Geometry: final body of the model. Coordinates: model frame, mm. Face numbers are marked on the shaded views. A direction names the side the tool comes from. Give positions to 0.01 mm unless a question says otherwise; leave off trailing zeros. Order: outer loops, then holes, each group sorted by start corner. A loop starts at its lowest first (then second) coordinate and runs counter-clockwise, first axis right, second up. Notation, with made-up numbers: (68.5, -38) - (106.5, -38) arc R20 cw to (106.5, -26) - close; hole circle Ø7 at (14.5, -37). An arc over 180 degrees is marked (long way). One line per item, written item: value.
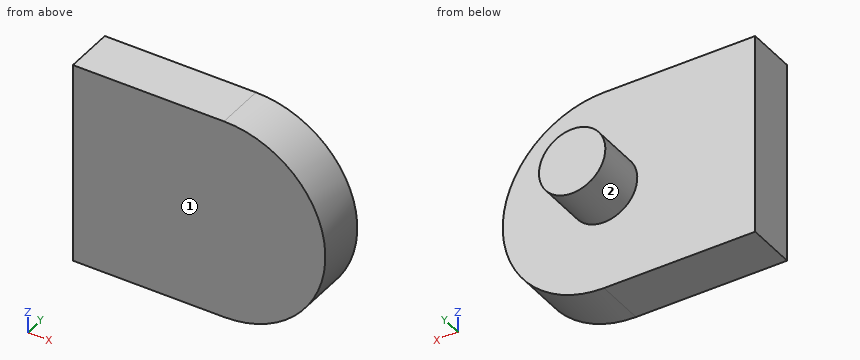
```python
from build123d import *

# Parameters (mm, degrees)
BOSS_EXTRUDE1_DEPTH = 3
SKETCH4_R           = 2
BOSS_EXTRUDE2_DEPTH = 3


with BuildPart() as part:
    # Sketch3 → Boss-Extrude1 (new body)
    with BuildSketch(Plane(origin=(0, 0, 0), x_dir=(1, 0, 0), z_dir=(0, 1, 0))):
        with BuildLine():
            Line((-20.336842105, 8.293859649), (-11.236842105, 8.293859649))
            ThreePointArc((-11.236842105, 8.293859649), (-5.136842105, 2.193859649), (-11.236842105, -3.906140351))
            Line((-11.236842105, -3.906140351), (-20.336842105, -3.906140351))
            Line((-20.336842105, -3.906140351), (-20.336842105, 8.293859649))
        make_face()
    extrude(amount=BOSS_EXTRUDE1_DEPTH)

    # Sketch4 → Boss-Extrude2 (add)
    with BuildSketch(Plane(origin=(0, 3, 0), x_dir=(1, 0, 0), z_dir=(0, 1, 0))):
        with Locations(Location((-11.236842105, 2.193859649, 0), (0, 0, 270))):
            Circle(SKETCH4_R)
    extrude(amount=BOSS_EXTRUDE2_DEPTH)


solid = part.part
```
1) Section A-A, the plane z = -3. Return loops of the section in (x, y), then the cut area to 3 significant figures.
Answers below:
outline: (-20.34, 0) - (-5.19, 0) - (-5.19, 3) - (-9.41, 3) - (-9.41, 6) - (-13.07, 6) - (-13.07, 3) - (-20.34, 3) - close
area: 56.4 mm^2
2) Set-up query: the marked faces 1 and 2. Return all of +Z, -Z, +X, -X, +Y, -Y with unobstructed straight access to the full face (end or side cutting, diameter ignored); none if empty.
Answers below:
face 1: +Z, -Z, +X, -X, -Y
face 2: +Y
3) Section C-C, the plane x = -18.5. Return loops of the section in (y, z).
Answers below:
outline: (0, -8.29) - (3, -8.29) - (3, 3.91) - (0, 3.91) - close
4) Material intervals for line 1 along Y through (x, z) = (-7.25, -4.5); line 2 along X through (y, z) = (2.85, -2); line 3 along Z through (x, y) = (-11.75, 4.15), sorted ascending.
Answers below:
line 1: 0 to 3
line 2: -20.34 to -5.14
line 3: -4.13 to -0.26
5) First-contact query: pin 1 (4 mm diameter, centred on x = -10, z = 1.5, fed in from -Y). Flat tip, straight axial feed; report the tip coordinate or a pass-through.
Answers below:
pin 1: y = 0
6) Section B-B, the plane y = 1.35. Return loops of the section in (x, z).
Answers below:
outline: (-20.34, -8.29) - (-11.24, -8.29) arc R6.1 ccw to (-11.24, 3.91) - (-20.34, 3.91) - close
7) Section D-D, the plane y = 4. Return loops of the section in (x, z), then the cut area to 3 significant figures.
Answers below:
outline: circle Ø4 at (-11.24, -2.19)
area: 12.6 mm^2
